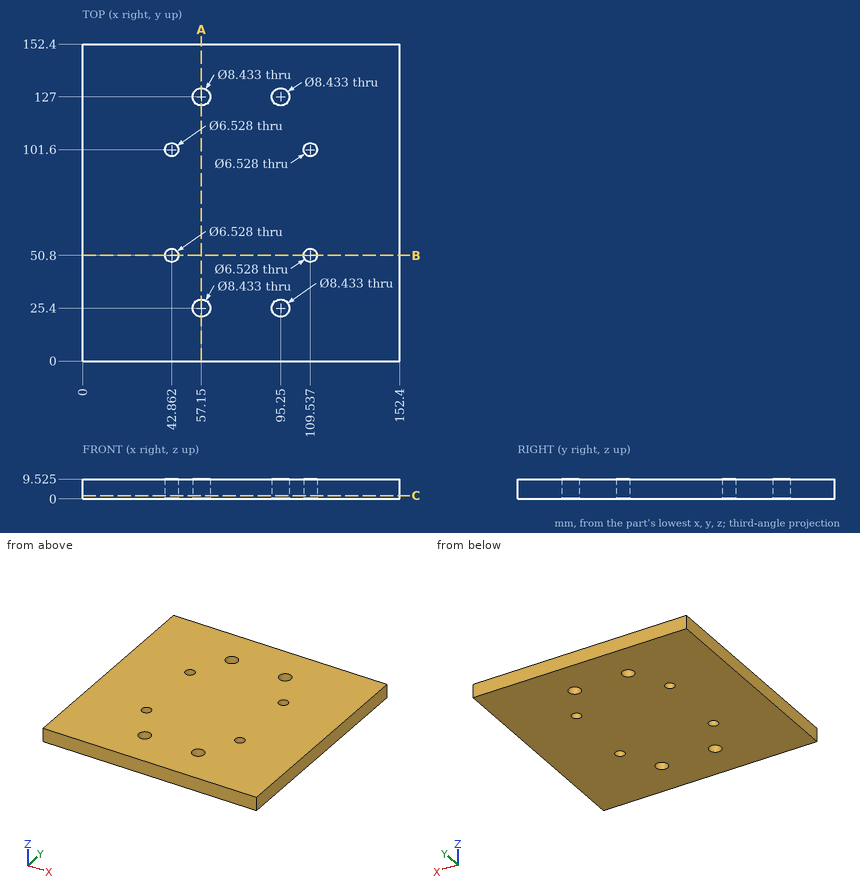
Input: dimensioned drawing with shaded views. Units: mm. Origin: part minimum x, y, z. Coordinates: 2 decimals unless noted, no trailing zeros. Order: outer loops, then holes, each group sorted by start corner. A loop starts at its lowest first (then second) coordinate and runs counter-clockwise, first axis right, second up. Notation, with made-up numbers: (44.5, 32.5) -> (94.5, 32.5) arc R19 cw to (94.5, 68.5) -> close; hole circle Ø9 at (-10.5, -30). An arc over 180 degrees is marked (long way). Use CSV: the item, a comma, the result in double quotes.
1) Pin query (flat end, axial travel): pin 1 Ø8.5 at (x, y) = (109.54, 50.8) entering from -Z. Return the tip coordinate at first contact, or that it passes through.
Findings:
pin 1,"stops at z = 0"
2) Section A-A on x = 57.15. Output: boundary loops of the cut face in (y, z) (1 decimal), then the cut area to 3 significant figures.
Findings:
outline,"(0, 0) -> (21.2, 0) -> (21.2, 9.5) -> (0, 9.5) -> close; (29.6, 0) -> (122.8, 0) -> (122.8, 9.5) -> (29.6, 9.5) -> close; (131.2, 0) -> (152.4, 0) -> (152.4, 9.5) -> (131.2, 9.5) -> close"
area,"1,290 mm^2"
3) Line query: line 1 (Y direction, x = 57.15, z = 7.25); line 2 (Y direction, x = 44.5, z = 3.25) (1 decimal); line 3 (X direction, y = 102.5, z = 4) (1 decimal). Output: solid intervals per line, ascending.
Findings:
line 1,"y = 0 to 21.18, 29.62 to 122.78, 131.22 to 152.4"
line 2,"y = 0 to 48, 53.6 to 98.8, 104.4 to 152.4"
line 3,"x = 0 to 39.7, 46 to 106.4, 112.7 to 152.4"
4) Section B-B on y = 50.8. Output: boundary loops of the cut face in (x, z) (1 decimal), then the cut area to 3 significant figures.
Findings:
outline,"(0, 0) -> (39.6, 0) -> (39.6, 9.5) -> (0, 9.5) -> close; (46.1, 0) -> (106.3, 0) -> (106.3, 9.5) -> (46.1, 9.5) -> close; (112.8, 0) -> (152.4, 0) -> (152.4, 9.5) -> (112.8, 9.5) -> close"
area,"1,330 mm^2"
5) Section C-C on z = 1.5. State how many separate pieces and enclosed holes the cut face has, then the cut area to 3 significant figures.
Findings:
separate pieces,"1"
enclosed holes,"8"
area,"22,900 mm^2"
